from build123d import *

# Parameters (mm, degrees)
BOSS_EXTRUDE1_DEPTH = 20
SKETCH2_R           = 13
CUT_EXTRUDE1_DEPTH  = 40


with BuildPart() as part:
    # Sketch1 → Boss-Extrude1 (new, symmetric)
    with BuildSketch(Plane.XY):
        Polygon((0, 0), (0, 14), (-8, 14), (-8, 64), (10, 64), (10, 10), (29, 10), (29, 25), (39, 25), (39, 0), align=None)
    extrude(amount=BOSS_EXTRUDE1_DEPTH, both=True)

    # Sketch2 → Cut-Extrude1 (cut)
    with BuildSketch(Plane(origin=(10, 0, 0), x_dir=(0, 0, -1), z_dir=(1, 0, 0))):
        with Locations(Location((0, 44, 0), (0, 0, 90))):
            Circle(SKETCH2_R)
    extrude(amount=-CUT_EXTRUDE1_DEPTH, mode=Mode.SUBTRACT)


solid = part.part
Input: part model. Units: mm. Frame: model coordinates. A direction names the side the tool comes from. Coordinates: 2 decimals unless noted, no trailing zeros. Loops run counter-clockwise (first coordinate to the right, second up) from the corner with the lowest first, then second, coordinate; pieces in that order, holes last.
(1) Section D-D on y = 15. Return the cut outline in (x, z), then the cut area to 3 significant figures.
(2) First-contact query: pin 1 Ø8 at (x, z) = (5.5, 8.5) entering from -Y; pin 2 Ø8 at (x, z) = (33.5, 2.5) entering from +Y; pin 3 Ø20 at (y, z) = (36, 1) entering from +X; pin 4 Ø12 at (x, z) = (18, -1.5) entering from +Y. Flat tips, straight axial feed; report the tip coordinate or a pass-through.
(3) Section C-C on x = -4.5. Return the cut outline in (y, z).
(4) Section B-B on z = 0. Return the cut outline in (x, y), then the cut area to 3 significant figures.
(5) Section A-A on y = 44. Return the cut outline in (x, z).
(6) Pull-direction query (X, two-part tool) for faces 4 (the face through (0, 7, 0)), 5 (the face through (10, 31, -4)), 6 (the face through (-4, 14, 0)); classes: released by +X, released by -X, zero draft, split by the parting line, or undercut.
(7) Material intervals for probe 1 along X at (y, z) = (12, 15.5); probe 2 along Z at (x, y) = (4.5, 44); probe 3 along Y at (x, z) = (36.5, -13.5), sorted ascending.
(8) Set-up query: faces 1 (the face through (29, 17, 0)), 2 (the face through (-8, 28, 0)), 3 (the face through (34, 25, 0)). Return all of +Z, -Z, +X, -X, +Y, -Y with unobstructed straight access to the full face (end or side cutting, diameter ignored); none if empty.
Data:
1. outline: (-8, -20) - (10, -20) - (10, 20) - (-8, 20) - close; (29, -20) - (39, -20) - (39, 20) - (29, 20) - close
1. area: 1,120 mm2
2. pin 1: stops at y = 0
2. pin 2: stops at y = 25
2. pin 3: stops at x = 10
2. pin 4: stops at y = 10
3. outline: (14, -20) - (64, -20) - (64, 20) - (14, 20) - close; hole circle Ø26 at (44, 0)
4. outline: (-8, 14) - (0, 14) - (0, 0) - (39, 0) - (39, 25) - (29, 25) - (29, 10) - (10, 10) - (10, 31) - (-8, 31) - close; (-8, 57) - (10, 57) - (10, 64) - (-8, 64) - close
4. area: 1,010 mm2
5. outline: (-8, -20) - (10, -20) - (10, -13) - (-8, -13) - close; (-8, 13) - (10, 13) - (10, 20) - (-8, 20) - close
6. face 4: released by -X
6. face 5: undercut
6. face 6: zero draft
7. probe 1: x = 0 to 10, 29 to 39
7. probe 2: z = -20 to -13, 13 to 20
7. probe 3: y = 0 to 25
8. face 1: +Z, -Z, +Y
8. face 2: +Z, -Z, -X, +Y, -Y
8. face 3: +Z, -Z, +X, +Y
